Autodesk Fusion 360 part; units mm, degrees
sketch "Bottom Part" plane through (0, 0, 0) normal (0, 1, 0) x (1, 0, 0)
  line L0 (-57, -32) -> (57, -32)
  line L1 (57, 32) -> (-57, 32)
  circle A0 centre (57, 0) radius 11
  circle A1 centre (-57, 0) radius 11
  arc A2 (-57, 32) -> (-57, -32) centre (-57, 0) ccw
  arc A3 (-57, 32) -> (-57, -32) centre (-57, 0) ccw
  arc A4 (57, -32) -> (57, 32) centre (57, 0) ccw
  dimension "d1" = 114
  dimension "d2" = 64
  dimension "d3" = 32
  dimension "d4" = 32
  dimension "d5" = 22
  dimension "d6" = 22
extrude "Extrude1" add sketch "Bottom Part" along normal blind 19
sketch "Vertical Part" plane through (0, 19, 0) normal (0, 1, 0) x (-1, 0, 0)
  circle A0 centre (57, 0) radius 11
  circle A1 centre (-57, 0) radius 11
  arc A2 (-57, 32) -> (-57, -32) centre (-57, 0) ccw
  line L0 (-57, -32) -> (57, -32)
  arc A3 (57, -32) -> (57, 32) centre (57, 0) ccw
  line L1 (57, 32) -> (-57, 32)
  line L2 (-32, -32) -> (32, -32)
  line L3 (32, -32) -> (32, 32)
  line L4 (32, 32) -> (-32, 32)
  line L5 (-32, 32) -> (-32, -32)
  line L6 (-32, -32) -> (32, 32) construction
  line L7 (32, -32) -> (-32, 32) construction
  line L8 (19, 32) -> (-19, 32)
  line L9 (-19, 32) -> (-19, -19)
  line L10 (-19, -19) -> (19, -19)
  line L11 (19, -19) -> (19, 32)
  dimension "d9" = 64
  dimension "d10" = 64
  dimension "d11" = 38
  dimension "d12" = 51
  dimension "d13" = 13
extrude "Extrude2" add sketch "Vertical Part" along normal blind 45 contours L1 L4 L8 L9 L10 L11
chamfer "Chamfer2" distance 51 distance2 45 1 edges at (0, 64, 32) measured on face at (6.3333, 64, 15)
extrude "Extrude4" add sketch "Vertical Part" along normal blind 45 contours L0 L1 L2 L3 L4 L5 L9 L10 L11
equation "d14 = 64 mm - 19 mm"
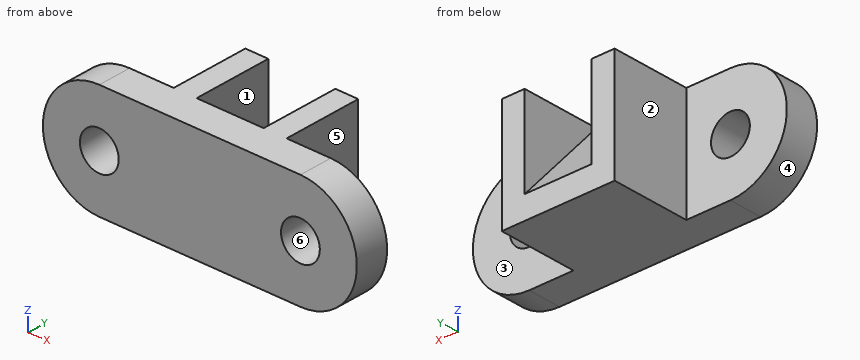
Geometry: final body of the model. Coordinates: model frame, mm. Face numbers are marked on the shaded views. A direction names the side the tool comes from. Round coordinates to 2 decimals unless told otherwise and drop trailing zeros. Order: outer loops, then holes, each group sorted by start corner. A loop starts at its lowest first (then second) coordinate and runs counter-clockwise, first axis right, second up. Notation, with made-up numbers: (30.25, 1.5) - (41.25, 1.5) arc R23 ccw to (41.25, 27.5) - close; hole circle Ø6 at (79, 13.5). An arc over 180 degrees is marked (long way). Write each question's results on one line, items separated by ' | '.
Item 1: Reachability of the marked faces 1, 2 and 3 from +Z, -Z, +X, -X, +Y, -Y: full face, straight path, thin tool, end or side. Return the list, or none.
Completed:
face 1: +Z, +Y | face 2: +Z, -Z, -X, +Y | face 3: +Z, -Z, +X, +Y
Item 2: First-contact query: pin 1 Ø2 at (y, z) = (35, 25) entering from -X; pin 2 Ø17 at (x, z) = (74.5, 3.5) entering from +Y; pin 3 Ø10 at (y, z) = (47, -16.5) entering from +X. Flat tips, straight axial feed; report the tip coordinate or a pass-through.
Completed:
pin 1: x = -32 | pin 2: y = 19 | pin 3: x = 32
Item 3: Section B-B, the plane z = -8. Return the cut outline in (x, y).
Completed:
outline: (-87.98, 0) - (-64.55, 0) - (-64.55, 19) - (-87.98, 19) - close; (-49.45, 0) - (49.45, 0) - (49.45, 19) - (32, 19) - (32, 64) - (19, 64) - (19, 54.3) - (-19, 54.3) - (-19, 64) - (-32, 64) - (-32, 19) - (-49.45, 19) - close; (64.55, 0) - (87.98, 0) - (87.98, 19) - (64.55, 19) - close
Item 4: Material intervals for line 1 along X through (y, z) = (11, 0); line 2 along Z through (x, y) = (57, 15.25); line 3 along X through (y, z) = (59.5, 17.5), sorted ascending. Write a range as [from, to].
Completed:
line 1: [-89, -68], [-46, 46], [68, 89] | line 2: [-32, -11], [11, 32] | line 3: [-32, -19], [19, 32]
Item 5: Section C-C, the plane x = 51. Return the cut outline in (y, z).
Completed:
outline: (0, -32) - (19, -32) - (19, -9.22) - (0, -9.22) - close; (0, 9.22) - (19, 9.22) - (19, 32) - (0, 32) - close
Item 6: Section D-D, the plane y = 39. Return the cut outline in (x, z).
Completed:
outline: (-32, -32) - (32, -32) - (32, 32) - (19, 32) - (19, 9.34) - (-19, 9.34) - (-19, 32) - (-32, 32) - close
Item 7: Section A-A, the plane y = 10.5. Return the cut outline in (x, z), and give its area (3 significant figures).
Completed:
outline: (-57, -32) - (57, -32) arc R32 ccw to (57, 32) - (-57, 32) arc R32 ccw to start; hole circle Ø22 at (-57, 0); hole circle Ø22 at (57, 0) | area: 9,750 mm^2
Item 8: Mould query, pull axis Z, two halves, no side actions, for the marked faces 4, 5 and 6. Classes: pulls with the +Z half, pulls with the -Z half, needs draft (parallel to the pull), parting line crosses it, or undercut.
Completed:
face 4: parting line crosses it | face 5: needs draft | face 6: undercut
